from build123d import *

# Parameters (mm, degrees)
F0_R     = 6.35
F1_DEPTH = 152.4
F2_T     = -2.54
F3_W     = 248.92
F3_H     = 147.32
F4_DEPTH = 25.4
F5_W     = 71.842049
F5_H     = 147.32
F6_DEPTH = 25.4


with BuildPart() as f1:
    # F0 (on Front) → F1 (new body)
    with BuildSketch(Plane.XZ):
        Polygon((-76.2, 95.25), (-127, 44.45), (-127, 0), (127, 0), (127, 44.45), (76.2, 95.25), align=None)
        with Locations((-101.6, 12.7)):
            Circle(F0_R, mode=Mode.SUBTRACT)
        with Locations((101.6, 12.7)):
            Circle(F0_R, mode=Mode.SUBTRACT)
    extrude(amount=F1_DEPTH)

    # F2
    f2_openings = [f1.faces().sort_by_distance(p)[0] for p in [
        (0, -76.2, 0),
    ]]
    offset(amount=F2_T, openings=f2_openings)

    # F3 (on face) → F4 (cut)
    with BuildSketch(Plane(origin=(0, 0, 0), x_dir=(1, 0, 0), z_dir=(0, 0, -1))):
        with Locations((0, 76.2)):
            Rectangle(F3_W, F3_H)
    extrude(amount=-F4_DEPTH, mode=Mode.SUBTRACT)

    # F5 (on face) → F6 (cut)
    with BuildSketch(Plane(origin=(85.725, 0, 85.725), x_dir=(0.707107, 0, -0.707107), z_dir=(0.707107, 0, 0.707107))):
        with Locations((22.45064, -76.2)):
            Rectangle(F5_W, F5_H)
    extrude(amount=-F6_DEPTH, mode=Mode.SUBTRACT)


solid = f1.part
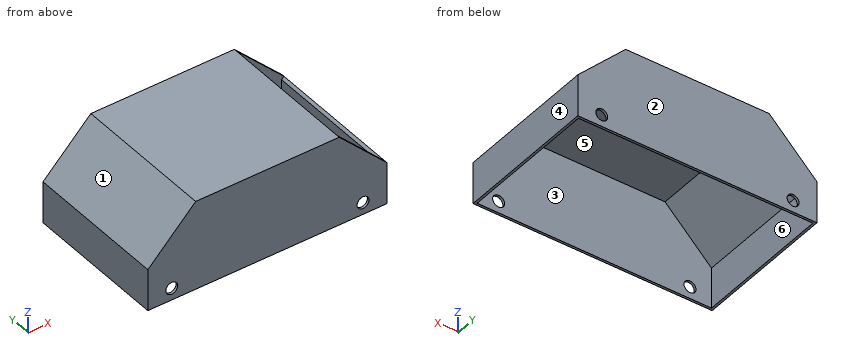
Build history of the part. All positions in model axes, mm. Face numbers are marked on the shaded views. A direction names the side the tool comes from. Round coordinates to 2 decimals unless told otherwise and drop trailing zeros. Write each loop counter-clockwise with the first axis right and the second up, starting at its lowest first coordinate (ties: lowest second). Pieces come first, ordered by that corner, then holes. Notation, with made-up numbers: (-37.5, 31) - (-24.5, 31) arc R31 cw to (-24.5, 61) - close; hole circle Ø7 at (88.25, 72). An arc over 180 degrees is marked (long way). Use CSV: the item, a comma, the result in double quotes.
(1) Band-saw the part on A-A (x = 85). Write the cut outline in (y, z), plus the area to 3 significant figures.
Response:
outline,"(-152.4, 0) - (-149.86, 0) - (-149.86, 86.45) - (-152.4, 86.45) - close; (-2.54, 0) - (0, 0) - (0, 86.45) - (-2.54, 86.45) - close"
area,"439 mm²"
(2) 3-axis set-ups, long thin cutter, end or side, ignore diameter. For the marked faces 4, 5 and 6: which of +Z, -Z, +X, -X, +Y, -Y reach the whole face in a straight line?
Response:
face 4,"+Z, -Z, +X, +Y, -Y"
face 5,"-Z, +X"
face 6,"-Z"
(3) Pin check, flat tips, straight feed: P1, Ø10, axis at x = 1, y = -68, coming from the -Z side; P2, Ø7.5, axis at x = 101.6, z = 12.7, coming from the +Y side. Stop position of each tip, or through.
Response:
P1,"z = 92.71"
P2,"through"
(4) Band-saw the part on D-D (z = 26.5). Write the cut outline in (x, y).
Response:
outline,"(-127, -152.4) - (127, -152.4) - (127, 0) - (-127, 0) - close; hole (-124.46, -149.86) - (124.46, -149.86) - (124.46, -2.54) - (-124.46, -2.54) - close"
(5) Band-saw the part on C-C (z = 12.7). Write the cut outline in (x, y).
Response:
outline,"(-127, -152.4) - (-107.95, -152.4) - (-107.95, -149.86) - (-124.46, -149.86) - (-124.46, -2.54) - (-107.95, -2.54) - (-107.95, 0) - (-127, 0) - close; (-95.25, -152.4) - (95.25, -152.4) - (95.25, -149.86) - (-95.25, -149.86) - close; (-95.25, -2.54) - (95.25, -2.54) - (95.25, 0) - (-95.25, 0) - close; (107.95, -152.4) - (127, -152.4) - (127, 0) - (107.95, 0) - (107.95, -2.54) - (124.46, -2.54) - (124.46, -149.86) - (107.95, -149.86) - close"
(6) Band-saw the part on B-B (y = -76). Write the cut outline in (x, z), plus the area to 3 significant figures.
Response:
outline,"(-127, 0) - (-124.46, 0) - (-124.46, 43.4) - (-75.15, 92.71) - (73.66, 92.71) - (76.2, 95.25) - (-76.2, 95.25) - (-127, 44.45) - close; (124.46, 0) - (127, 0) - (127, 44.45) - (124.46, 41.91) - close"
area,"784 mm²"
(7) Mould opens along X. For the marked faces 1, 2 and 3 say: pulls with the +X half, pulls with the -X half, needs draft (parallel to the pull), parting line crosses it, or undercut.
Response:
face 1,"pulls with the -X half"
face 2,"needs draft"
face 3,"undercut"
(8) Wall check: line 1 (X direction, y = -1, z = 12); line 2 (Y direction, x = 4.5, z = 91.5); line 3 (X direction, y = -34.5, z = 6). Give the ranges that are in metal, low to high.
Response:
line 1,"-127 to -107.91, -95.29 to 95.29, 107.91 to 127"
line 2,"-152.4 to -149.86, -2.54 to 0"
line 3,"-127 to -124.46, 124.46 to 127"
